Here's how the part is built. I have some questions about the finished solid (model axes, mm). Coordinates: 2 decimals unless noted, no trailing zeros. Loops run counter-clockwise (first coordinate to the right, second up) from the corner with the lowest first, then second, coordinate; pieces in that order, holes last. Notation, with made-up numbers: (86, -17.5) - (125, -17.5) arc R33 ccw to (125, 18.5) - close; hole circle Ø3 at (25.25, -35). An arc over 180 degrees is marked (long way). Use a Markdown table: item, result.
```python
from build123d import *

# Parameters (mm, degrees)
SCHIZZO1_W                   = 420
SCHIZZO1_H                   = 45.92
PIASTRABASE_DEPTH            = 2
SCHIZZO2_R                   = 9
FOROTUBOMOTORE_DEPTH         = 212.260885163
ESTRUSIONE_ESTRUSIONE1_DEPTH = 2


with BuildPart() as part:
    # Schizzo1 → PiastraBase (new body)
    with BuildSketch(Plane.XY):
        Rectangle(SCHIZZO1_W, SCHIZZO1_H)
    extrude(amount=PIASTRABASE_DEPTH)

    # Schizzo2 → ForoTuboMotore (cut, through all)
    with BuildSketch(Plane.XY.offset(2)):
        with Locations((-140.833333333, 2.04)):
            Circle(SCHIZZO2_R)
    forotubomotore = extrude(amount=-FOROTUBOMOTORE_DEPTH, mode=Mode.SUBTRACT)

    # Specchia1: ForoTuboMotore across plane
    add(forotubomotore.mirror(Plane(origin=(0, 0, 0), x_dir=(0, 0, 1), z_dir=(1, 0, 0))), mode=Mode.SUBTRACT)

    # Schizzo4 → Estrusione-Estrusione1 (add)
    with BuildSketch(Plane.XY.offset(2)):
        Polygon((104.844657179, 22.96), (0, 29.70924382), (0, 22.96), align=None)
    estrusione_estrusione1 = extrude(amount=-ESTRUSIONE_ESTRUSIONE1_DEPTH)

    # Specchia2: Estrusione-Estrusione1 across plane
    add(estrusione_estrusione1.mirror(Plane(origin=(0, 0, 0), x_dir=(0, 0, 1), z_dir=(1, 0, 0))))


solid = part.part
```
Q1. I want a section at C-C, the plane x = 173. Write out the boundary of the cut face in (y, z).
Check values:
| item | result |
|---|---|
| outline | (-22.96, 0) - (22.96, 0) - (22.96, 2) - (-22.96, 2) - close |
Q2. If we mould it in two halves opening along X, with no side actions, what happens to faces 1 (the face through (3, 4, 2)), 2 (the face through (53.156, 26.287, 1.014)), 3 (the face through (-149.825, 2.436, 1.014))? For each: pulls with the +X half, pulls with the -X half, needs draft (parallel to the pull), parting line crosses it, or undercut.
Check values:
| item | result |
|---|---|
| face 1 | needs draft |
| face 2 | pulls with the +X half |
| face 3 | undercut |
Q3. I want a section at D-D, the plane x = -34. Write out the boundary of the cut face in (y, z), then the cut area to 3 significant figures.
Check values:
| item | result |
|---|---|
| outline | (-22.96, 0) - (27.52, 0) - (27.52, 2) - (-22.96, 2) - close |
| area | 101 mm^2 |
Q4. Please list where these lines run through material, in increasing order: L1, parallel to X at y = -5.5, z = 1.3; L2, parallel to Y at x = -191.5, z = 0.4; L3, parallel to X at y = -4.5, z = 1.9. Write a range as from..to.
Check values:
| item | result |
|---|---|
| L1 | -210..-145.75, -135.92..135.92, 145.75..210 |
| L2 | -22.96..22.96 |
| L3 | -210..-147.02, -134.65..134.65, 147.02..210 |
Q5. I want a section at A-A, the plane y = 2.04. Write out the boundary of the cut face in (x, z).
Check values:
| item | result |
|---|---|
| outline | (-210, 0) - (-149.83, 0) - (-149.83, 2) - (-210, 2) - close; (-131.83, 0) - (131.83, 0) - (131.83, 2) - (-131.83, 2) - close; (149.83, 0) - (210, 0) - (210, 2) - (149.83, 2) - close |
Q6. Will this pin go through, and if not, where does the flat tip stop? P1, Ø1, axis at x = 163, z = 1, coming from the +Y side.
Check values:
| item | result |
|---|---|
| P1 | y = 22.96 |
Q7. I want a section at B-B, the plane z = 0.6. Write out the boundary of the cut face in (x, y).
Check values:
| item | result |
|---|---|
| outline | (-210, -22.96) - (210, -22.96) - (210, 22.96) - (104.84, 22.96) - (0, 29.71) - (-104.84, 22.96) - (-210, 22.96) - close; hole circle Ø18 at (-140.83, 2.04); hole circle Ø18 at (140.83, 2.04) |
